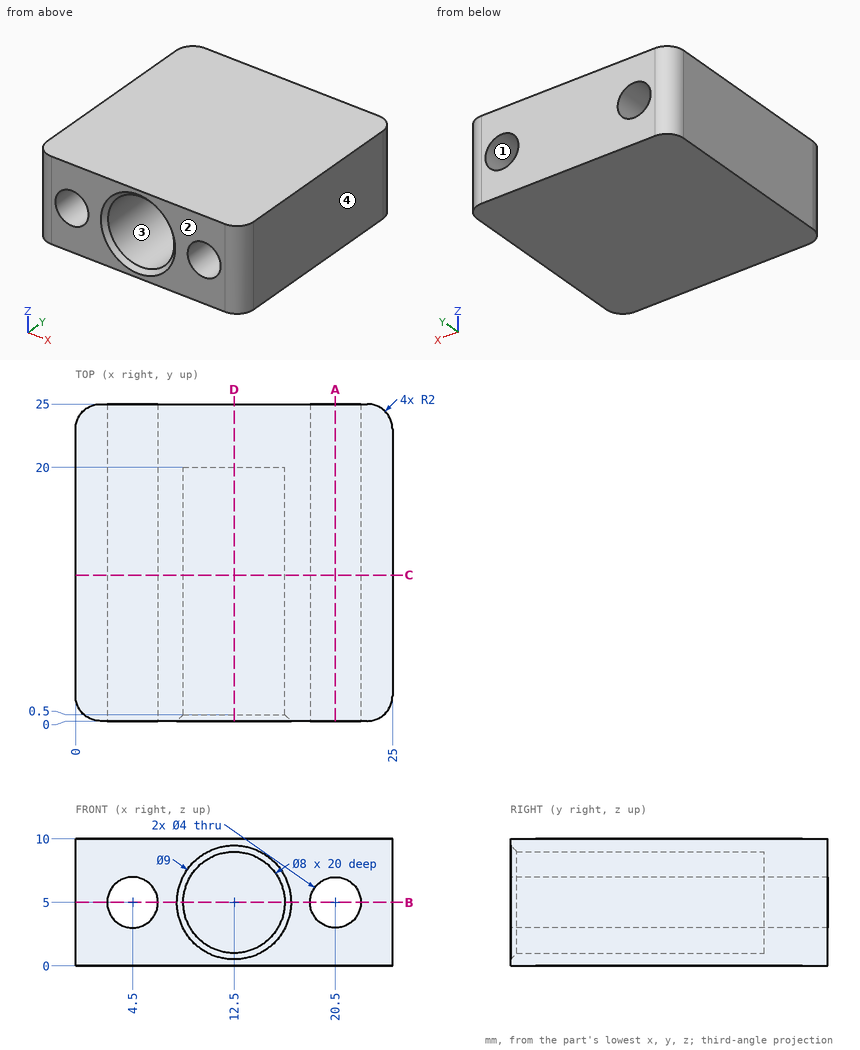
Job drawing, mm, ordinate dimensions from the low corner. One solid piece. Round coordinates to 2 decimals unless told otherwise and drop trailing zeros. Order: outer loops, then holes, each group sorted by start corner. A loop starts at its lowest first (then second) coordinate and runs counter-clockwise, first axis right, second up. Notation, with made-up numbers: (2, 53.5) - (22, 53.5) arc R11 ccw to (22, 74.5) - close; hole circle Ø3 at (12, 71.5). An arc over 180 degrees is marked (long way). Use CSV: the item, a comma, the result in double quotes. Start each with the question number.
1) Two-plate mould, pull along X, no slides. Class the marked faces 1, 2, 3 and 4: pulls with the +X half, pulls with the -X half, needs draft (parallel to the pull), parting line crosses it, or undercut.
2) Saw through at B-B (z = 5). List the corners of the cut face in (x, y).
3) Saw through at D-D (x = 12.5). List the corners of the cut face in (y, z), and give its area (4 significant figures).
4) Pin check, flat tip, straight feed: pin 1 Ø4 at (x, z) = (10.5, 4) entering from -Y. Stop position of the tip, or through.
5) Saw through at A-A (x = 20.5). List the corners of the cut face in (y, z), and give its area (3 significant figures).
6) Saw through at C-C (y = 11.5). List the corners of the cut face in (x, z).
7) Wall check: L1, parallel to X at y = 9.75, z = 5; L2, parallel to Z at x = 12.5, y = 14.25; L3, parallel to X at y = 5, z = 5.5. Give the ranges that are in metal, low to high. Write a range as [from, to].
Values follow:
1,face 1,"undercut"
1,face 2,"needs draft"
1,face 3,"undercut"
1,face 4,"pulls with the +X half"
2,outline,"(0, 2) arc R2 ccw to (2, 0) - (2.5, 0) - (2.5, 25) - (2, 25) arc R2 ccw to (0, 23) - close; (6.5, 0) - (8, 0) - (8.5, 0.5) - (8.5, 20) - (16.5, 20) - (16.5, 0.5) - (17, 0) - (18.5, 0) - (18.5, 25) - (6.5, 25) - close; (22.5, 0) - (23, 0) arc R2 ccw to (25, 2) - (25, 23) arc R2 ccw to (23, 25) - (22.5, 25) - close"
3,outline,"(0, 0) - (25, 0) - (25, 10) - (0, 10) - (0, 9.5) - (0.5, 9) - (20, 9) - (20, 1) - (0.5, 1) - (0, 0.5) - close"
3,area,"89.75 mm2"
4,pin 1,"stops at y = 0.26"
5,outline,"(0, 0) - (25, 0) - (25, 3) - (0, 3) - close; (0, 7) - (25, 7) - (25, 10) - (0, 10) - close"
5,area,"150 mm2"
6,outline,"(0, 0) - (25, 0) - (25, 10) - (0, 10) - close; hole circle Ø4 at (4.5, 5); hole circle Ø8 at (12.5, 5); hole circle Ø4 at (20.5, 5)"
7,L1,"x = [0, 2.5], [6.5, 8.5], [16.5, 18.5], [22.5, 25]"
7,L2,"z = [0, 1], [9, 10]"
7,L3,"x = [0, 2.56], [6.44, 8.53], [16.47, 18.56], [22.44, 25]"
